from build123d import *

# Parameters (mm, degrees)
RESSALTO_EXTRUS_O1_DEPTH = 6


with BuildPart() as part:
    # Esboço1 → Ressalto-extrusão1 (new body)
    with BuildSketch(Plane(origin=(0, 0, 0), x_dir=(1, 0, 0), z_dir=(0, 1, 0))):
        with BuildLine():
            Line((-4.233916189, 19.955016117), (355.507733721, 89.136102639))
            ThreePointArc((355.507733721, 89.136102639), (357.907745838, 88.272697698), (358.301043932, 85.75260983))
            Line((358.301043932, 85.75260983), (330, 15))
            Line((330, 15), (330, 0))
            Line((330, 0), (310, 0))
            Line((310, 0), (310, 15))
            Line((310, 15), (175, 15))
            Line((175, 15), (175, 0))
            Line((175, 0), (155, 0))
            Line((155, 0), (155, 15))
            Line((155, 15), (20, 15))
            Line((20, 15), (20, 0))
            Line((20, 0), (0, 0))
            Line((0, 0), (0, 15))
            Line((0, 15), (-3.761797705, 15))
            ThreePointArc((-3.761797705, 15), (-6.250526326, 17.262871653), (-4.233916189, 19.955016117))
        make_face()
    extrude(amount=RESSALTO_EXTRUS_O1_DEPTH)


solid = part.part
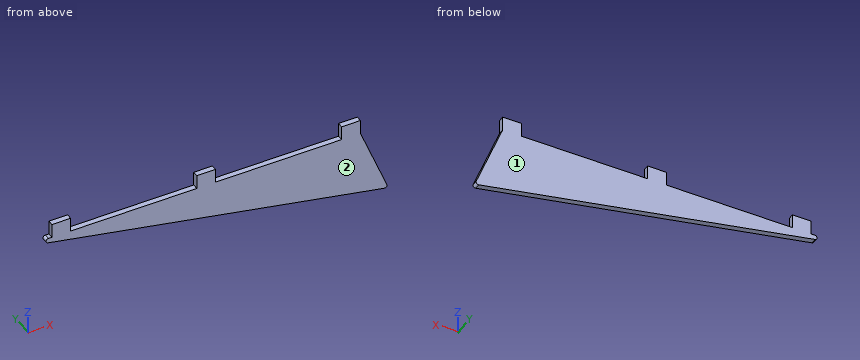
The listing builds one solid part. Answer for the finished solid, in the listing's coordinates (mm). Face numbers are marked on the shaded views. Coordinates: 2 decimals unless noted, no trailing zeros. Order: outer loops, then holes, each group sorted by start corner. A loop starts at its lowest first (then second) coordinate and runs counter-clockwise, first axis right, second up.
Q1. A cutting plane is placed at A-A, the plane y = 1.3. Write down the section's boundary in (x, z), and give its area (3 significant figures).
Q2. Given P1, Ø1.8, axis at x = 54.5, y = 3.5, coming from the +Z side; P2, Ø1.8, axis at y = 3, z = -8.5, coming from the -X side; P3, Ø2, axis at x = 127, y = 4, coming from the -Z side, each flat-ended and moving along its own axis, determine where each tip first touches the part or whether it passes through.
Q3. For a pull along Y with two mould halves and no side action, classify the marked faces 1 and 2 as pulls with the +Y half, pulls with the -Y half, needs draft (parallel to the pull), parting line crosses it, or undercut.
Q4. A cutting plane is placed at B-B, the plane z = -62. Write down the section's boundary in (x, y).
Q5. A cutting plane is placed at C-C, the plane x = 220. Write down the section's boundary in (y, z).
Q6. Consider line 1 (X direction, y = 2.1, z = -11); line 2 (Z direction, x = 79.5, y = 4.9); line 3 (Z direction, x = 120, y = 0.85). Determine where each line is inside the solid, lowest interval first.
Answers follow:
1. outline: (-4.23, -19.96) - (355.51, -89.14) arc R2.5 ccw to (358.3, -85.75) - (330, -15) - (330, 0) - (310, 0) - (310, -15) - (175, -15) - (175, 0) - (155, 0) - (155, -15) - (20, -15) - (20, 0) - (0, 0) - (0, -15) - (-3.76, -15) arc R2.5 ccw to start
1. area: 14,300 mm2
2. P1: stops at z = -15
2. P2: stops at x = 0
2. P3: stops at z = -45.38
3. face 1: pulls with the +Y half
3. face 2: pulls with the -Y half
4. outline: (214.4, 0) - (348.8, 0) - (348.8, 6) - (214.4, 6) - close
5. outline: (0, -63.08) - (6, -63.08) - (6, -15) - (0, -15) - close
6. line 1: x = 0 to 20, 155 to 175, 310 to 330
6. line 2: z = -36.06 to -15
6. line 3: z = -43.85 to -15
